Could you check a few things on this model? Use its own coordinates, in mm. A direction names the side the tool comes from. Round coordinates to 2 decimals unless told otherwise and drop trailing zeros. Loops run counter-clockwise (first coordinate to the right, second up) from the corner with the lowest first, then second, coordinate; pieces in that order, holes last. Notation, with made-up numbers: (77.5, 28) - (136.5, 28) arc R22 cw to (136.5, 56) - close; hole circle Ø6 at (-18.5, 76.25). An arc over 180 degrees is marked (long way). Use one line per item in the form item = value.
Autodesk Inventor part; units mm, degrees
ref_plane "YZ Plane" through (0, 0, 0) normal (1, 0, 0) x (0, 1, 0)
ref_plane "XZ Plane" through (0, 0, 0) normal (0, 1, 0) x (-1, 0, 0)
ref_plane "XY Plane" through (0, 0, 0) normal (0, 0, 1) x (1, 0, 0)
sketch "Sketch1" plane through (0, 0, 0) normal (0, 1, 0) x (-1, 0, 0)
  line L0 (0, 0) -> (80, 0)
  line L1 (80, 0) -> (80, -80)
  line L2 (80, -80) -> (0, -80)
  line L3 (0, -80) -> (0, 0)
  dimension "d0" = 80
  dimension "d1" = 80
extrude "Extrusion1" add sketch "Sketch1" along normal blind 10
sketch "Sketch2" plane through (0, 10, 0) normal (0, 1, 0) x (1, 0, 0)
  line L0 (-80, 0) -> (0, 0)
  line L1 (0, 0) -> (-80, 0)
  line L2 (-80, 0) -> (-80, 10)
  line L3 (-80, 10) -> (0, 10)
  line L4 (0, 10) -> (0, 0)
  line L5 (0, 80) -> (-80, 80)
  line L6 (-80, 0) -> (-70, 0)
  line L7 (-70, 0) -> (-70, 80)
  line L8 (-70, 80) -> (-80, 80)
  line L9 (-80, 80) -> (-80, 0)
  line L10 (-80, 80) -> (0, 80)
  line L11 (0, 80) -> (0, 70)
  line L12 (0, 70) -> (-80, 70)
  line L13 (-80, 70) -> (-80, 80)
  line L14 (0, 80) -> (-10, 80)
  line L15 (-10, 80) -> (-10, 0)
  line L16 (-10, 0) -> (0, 0)
  line L17 (0, 0) -> (0, 80)
  point P0 (-70, 10)
  point P1 (-70, 70)
  point P2 (-10, 70)
  point P3 (-10, 10)
  dimension "d4" = 10
  dimension "d5" = 10
  dimension "d6" = 10
  dimension "d7" = 10
  dimension "d8" = 80
  dimension "d9" = 0
extrude "Extrusion2" add sketch "Sketch2" along normal blind 80 contours L2 L3 L7 L0 | L7 L3 L15 L0 | L9 L12 L7 L3 | L15 L3 L4 L0 | L9 L5 L7 L12 | L15 L12 L17 L3 | L7 L5 L15 L12 | L15 L5 L11 L12
sketch "Sketch3" plane through (-80, 0, 0) normal (0, 0, 1) x (1, 0, 0)
  line L0 (10, 27) -> (22, 27)
  line L1 (22, 27) -> (22, 15)
  line L2 (22, 15) -> (10, 15)
  line L3 (10, 15) -> (10, 27)
  line L4 (0, 0) -> (0, 90)
  line L5 (0, 0) -> (80, 0)
  line L6 (58, 27) -> (70, 27)
  line L7 (70, 27) -> (70, 15)
  line L8 (70, 15) -> (58, 15)
  line L9 (58, 15) -> (58, 27)
  line L10 (80, 0) -> (80, 90)
  dimension "d12" = 12
  dimension "d13" = 12
  dimension "d14" = 10
  dimension "d15" = 15
  dimension "d16" = 12
  dimension "d17" = 12
  dimension "d18" = 10
  dimension "d19" = 15
sketch "Sketch4" plane through (0, 0, 0) normal (1, 0, 0) x (0, 0, -1)
  line L0 (10, 27) -> (22, 27)
  line L1 (22, 27) -> (22, 15)
  line L2 (22, 15) -> (10, 15)
  line L3 (10, 15) -> (10, 27)
  line L4 (0, 0) -> (0, 90)
  line L5 (0, 0) -> (80, 0)
  line L6 (58, 27) -> (70, 27)
  line L7 (70, 27) -> (70, 15)
  line L8 (70, 15) -> (58, 15)
  line L9 (58, 15) -> (58, 27)
  line L10 (80, 0) -> (80, 90)
  point P0 (16, 15)
  dimension "d20" = 12
  dimension "d21" = 12
  dimension "d22" = 10
  dimension "d23" = 15
  dimension "d24" = 12
  dimension "d25" = 12
  dimension "d26" = 10
  dimension "d27" = 15
sketch "Sketch5" plane through (0, 0, -80) normal (0, 0, -1) x (-1, 0, 0)
  line L0 (10, 27) -> (22, 27)
  line L1 (22, 27) -> (22, 15)
  line L2 (22, 15) -> (10, 15)
  line L3 (10, 15) -> (10, 27)
  line L4 (0, 0) -> (0, 90)
  line L5 (0, 0) -> (80, 0)
  line L6 (58, 27) -> (70, 27)
  line L7 (70, 27) -> (70, 15)
  line L8 (70, 15) -> (58, 15)
  line L9 (58, 15) -> (58, 27)
  line L10 (80, 0) -> (80, 90)
  dimension "d28" = 12
  dimension "d29" = 12
  dimension "d30" = 10
  dimension "d31" = 15
  dimension "d32" = 12
  dimension "d33" = 12
  dimension "d34" = 10
  dimension "d35" = 15
sketch "Sketch6" plane through (0, 0, -80) normal (0, 0, -1) x (-1, 0, 0)
  point P0 (0, 0)
sketch "Sketch7" plane through (-80, 0, -80) normal (-1, 0, 0) x (0, 0, 1)
  line L0 (10, 27) -> (22, 27)
  line L1 (22, 27) -> (22, 15)
  line L2 (22, 15) -> (10, 15)
  line L3 (10, 15) -> (10, 27)
  line L4 (0, 0) -> (0, 90)
  line L5 (0, 0) -> (80, 0)
  line L6 (58, 27) -> (70, 27)
  line L7 (70, 27) -> (70, 15)
  line L8 (70, 15) -> (58, 15)
  line L9 (58, 15) -> (58, 27)
  line L10 (80, 0) -> (80, 90)
  point P0 (16, 15)
  dimension "d36" = 12
  dimension "d37" = 12
  dimension "d38" = 10
  dimension "d39" = 15
  dimension "d40" = 12
  dimension "d41" = 12
  dimension "d42" = 10
  dimension "d43" = 15
extrude "Extrusion3" cut sketch "Sketch7" against normal blind 5
extrude "Extrusion4" cut sketch "Sketch4" against normal blind 5
extrude "Extrusion5" cut sketch "Sketch3" against normal blind 5
extrude "Extrusion6" cut sketch "Sketch5" against normal blind 5
properties part number "Box"
1. If we section it at B-B, the plane y = 33: Write out the boundary of the cut face in (x, z), plus the area to 3 significant figures.
Solution:
outline = (-80, -80) - (0, -80) - (0, 0) - (-80, 0) - close; hole (-70, -70) - (-10, -70) - (-10, -10) - (-70, -10) - close
area = 2,800 mm^2
2. If we section it at D-D, the plane x = -11.5: Write out the boundary of the cut face in (y, z), plus the area to 3 significant figures.
Solution:
outline = (0, -80) - (15, -80) - (15, -75) - (27, -75) - (27, -80) - (90, -80) - (90, -70) - (10, -70) - (10, -10) - (90, -10) - (90, 0) - (27, 0) - (27, -5) - (15, -5) - (15, 0) - (0, 0) - close
area = 2,280 mm^2
3. If we section it at A-A, the plane x = -52: Write out the boundary of the cut face in (y, z).
Solution:
outline = (0, -80) - (90, -80) - (90, -70) - (10, -70) - (10, -10) - (90, -10) - (90, 0) - (0, 0) - close
4. Please list where these lines run through material, in increasing order: line 1 along X through (y, z) = (66.5, -11.5); line 2 along Y through (x, z) = (-56, -61.5).
Solution:
line_1 = -80 to -70, -10 to 0
line_2 = 0 to 10
5. If we section it at C-C, the plane z = -60: Write out the boundary of the cut face in (x, y), plus the area to 3 significant figures.
Solution:
outline = (-80, 0) - (0, 0) - (0, 15) - (-5, 15) - (-5, 27) - (0, 27) - (0, 90) - (-10, 90) - (-10, 10) - (-70, 10) - (-70, 90) - (-80, 90) - (-80, 27) - (-75, 27) - (-75, 15) - (-80, 15) - close
area = 2,280 mm^2
6. On a 3-axis mill with a long thin cutter (end or side, diameter ignored), from which of +Z, -Z, +X, -X, +Y, -Y can I reach the whole of each face in a straight line? I mean faces 3 (the face through (-58, 21, -2)), 4 (the face through (-16, 15, -78)), 5 (the face through (-78, 15, -64)), 6 (the face through (-2, 27, -64)). Say none if no direction works.
Solution:
face_3 = +Z
face_4 = -Z
face_5 = -X
face_6 = +X
7. We'd pull the mould along Z, two halves only. Please class faces 1 (the face through (-22, 21, -2)), 2 (the face through (-5, 21, -16)): +Z half, -Z half, draft (parallel to the pull), parting line (faces both ways), or undercut.
Solution:
face_1 = draft
face_2 = undercut
8. For P1, Ø18, axis at x = -42, z = -42.5, coming from the +Y side, with a flat end and sliding along its axis, tell me the tip position at first contact or that it passes through.
Solution:
P1 = 10
